Source: three-view drawing plus pictorial views. Frame: mm from the lowest corner of the part. Give positions to 0.01 mm unless a question says otherwise; leave off trailing zeros. Loops run counter-clockwise (first coordinate to the right, second up) from the corner with the lowest first, then second, coordinate; pieces in that order, holes last. Notation, with made-up numbers: (-4, 24) - (38, 24) arc R26 ccw to (38, 47) - close; hole circle Ø9 at (45.5, -24.75). An arc over 180 degrees is marked (long way). Answer as a JSON object with one key per item and string values.
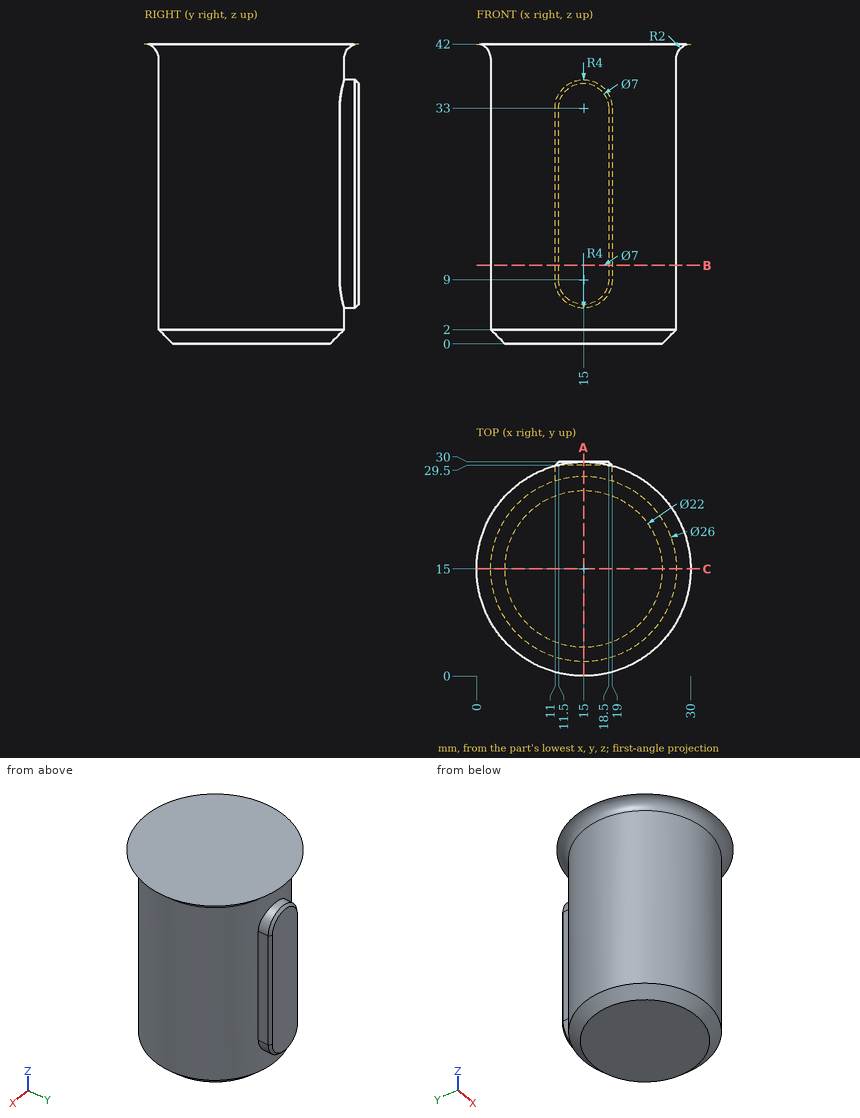
Item 1: Contact query for flat-ended pins moving along their axis: P1, Ø0.6, axis at y = 28, z = 16, coming from the -X side; P2, Ø1.1, axis at y = 28, z = 25.5, coming from the +X side; P3, Ø8, axis at y = 16, z = 7, coming from the -X side. Output: stop coordinate, or through.
Geometry check:
{"P1": "stops at x = 11", "P2": "stops at x = 19", "P3": "stops at x = 2"}
Item 2: Material intervals for line 1 (Y direction, x = 14.5, z = 40); line 2 (X direction, y = 27.75, z = 14); line 3 (Z direction, x = 25, y = 6.5), sorted ascending. Write a range as [from, to].
Geometry check:
{"line 1": "y = [2.01, 27.99]", "line 2": "x = [11, 19]", "line 3": "z = [40.69, 42]"}
Item 3: Cut plane B-B (z = 11). Return loops of the section in (x, y).
Geometry check:
{"outline": "(11, 27.37) arc R13 ccw (long way) to (19, 27.37) - (19, 29.5) - (18.5, 30) - (11.5, 30) - (11, 29.5) - close"}
Item 4: Cut plane A-A (x = 15). Return loops of the section in (y, z), then the cut area to 3 significant figures.
Geometry check:
{"outline": "(0, 42) arc R2 cw to (2, 40) - (2, 2) - (4, 0) - (26, 0) - (28, 2) - (28, 5) - (29.5, 5) - (30, 5.5) - (30, 36.5) - (29.5, 37) - (28, 37) - (28, 40) arc R2 cw to (30, 42) - close", "area": "1,150 mm2"}
Item 5: Cut plane C-C (y = 15). Return loops of the section in (x, z), then the cut area to 3 significant figures.
Geometry check:
{"outline": "(0, 42) arc R2 cw to (2, 40) - (2, 2) - (4, 0) - (26, 0) - (28, 2) - (28, 40) arc R2 cw to (30, 42) - close", "area": "1,090 mm2"}
